Autodesk Inventor part; units mm, degrees
ref_plane "Work Plane1" through (0, 304.8, 0) normal (0, -1, 0) x (1, 0, 0)
ref_plane "YZ Plane" through (0, 0, 0) normal (1, 0, 0) x (0, 1, 0)
ref_plane "XZ Plane" through (0, 0, 0) normal (0, 1, 0) x (-1, 0, 0)
sketch "Sketch1" plane through (0, 0, 0) normal (0, 0, 1) x (1, 0, 0)
  line L0 (0, 0) -> (1016, 0)
  line L1 (1016, 0) -> (1016, 609.6)
  line L2 (1016, 609.6) -> (0, 609.6)
  line L3 (0, 609.6) -> (0, 0)
  line L4 (12.7, 12.7) -> (1003.3, 12.7)
  line L5 (1003.3, 12.7) -> (1003.3, 596.9)
  line L6 (1003.3, 596.9) -> (12.7, 596.9)
  line L7 (12.7, 596.9) -> (12.7, 12.7)
  dimension "d0" = 609.6
  dimension "d1" = 1016
  dimension "d2" = 12.7
  dimension "d3" = 12.7
  dimension "d4" = 12.7
  dimension "d5" = 12.7
extrude "Extrusion1" add sketch "Sketch1" along normal blind 2032
extrude "Extrusion2" add sketch "Sketch1" along normal blind 12.7 contours L7 L6 L5 L4
ref_plane "Work Plane1" through (0, 304.8, 0) normal (0, -1, 0) x (1, 0, 0)
equation "\"d0\" = length"
equation "\"d1\" = width"
equation "\"d2\" = thickness"
equation "\"d3\" = thickness"
equation "\"d4\" = thickness"
equation "\"d5\" = thickness"
equation "\"d6\" = height"
equation "\"d8\" = thickness"
equation "\"length\" = 609.6"
equation "\"width\" = 1016"
equation "\"height\" = 2032"
equation "\"thickness\" = 12.7"
properties part number "box"
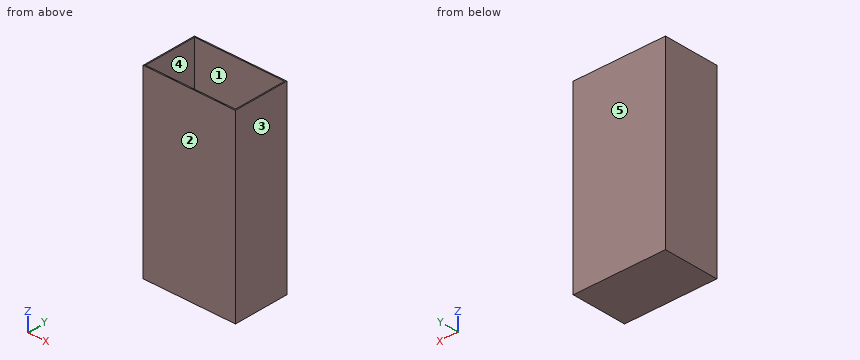
Could you check a few things on this model? Use its own coordinates, in mm. Face numbers are marked on the shaded views. A direction names the side the tool comes from. Coordinates: 2 decimals unless noted, no trailing zeros. Order: outer loops, then holes, each group sorted by start corner. A loop starts at its lowest first (then second) coordinate and runs counter-clockwise, first axis right, second up.
Q1. Will these pins go through, and if not, where does the flat tip stop? pin 1 (12 mm diameter, centred on x = 465.5, y = 282.5, fed in from +Z); pin 2 (3 mm diameter, centred on x = 151, y = 325.5, fed in from -Z).
Q2. Thinking about a two-plate mould opening in Y: for the marked faces 1, 2 and 3, which applies, released by +Y, released by -Y, zero draft, split by the parting line, or undercut?
Q3. Suppose I cut it at B-B on y = 64. Please give me the cut outline in (x, z), and give its area (3 significant figures).
Q4. Which directions (+Z, -Z, +X, -X, +Y, -Y) give clear straight access to the entire face, cutting with the end or side of a thin tool? Please do the marked faces 4 and 5.
Q5. Suppose I cut it at C-C on x = 803.5. Please give me the cut outline in (y, z), and give its area (3 significant figures).
Q6. Suppose I cut it at A-A on z = 1093.5. Please give me the cut outline in (x, y), and give its area (3 significant figures).
Q7. Please list where these lines run through material, in increasing order: L1, parallel to X at y = 469, z = 194; L2, parallel to Y at x = 709, z = 1917; L3, parallel to Z at x = 568.5, y = 299.
Answer:
1. pin 1: stops at z = 12.7
1. pin 2: stops at z = 0
2. face 1: undercut
2. face 2: released by -Y
2. face 3: zero draft
3. outline: (0, 0) - (1016, 0) - (1016, 2032) - (1003.3, 2032) - (1003.3, 12.7) - (12.7, 12.7) - (12.7, 2032) - (0, 2032) - close
3. area: 64,200 mm2
4. face 4: +Z
4. face 5: +Z, -Z, +X, -X, +Y
5. outline: (0, 0) - (609.6, 0) - (609.6, 2032) - (596.9, 2032) - (596.9, 12.7) - (12.7, 12.7) - (12.7, 2032) - (0, 2032) - close
5. area: 59,000 mm2
6. outline: (0, 0) - (1016, 0) - (1016, 609.6) - (0, 609.6) - close; hole (12.7, 12.7) - (1003.3, 12.7) - (1003.3, 596.9) - (12.7, 596.9) - close
6. area: 40,600 mm2
7. L1: x = 0 to 12.7, 1003.3 to 1016
7. L2: y = 0 to 12.7, 596.9 to 609.6
7. L3: z = 0 to 12.7
